Geometry: final body of the model. Coordinates: model frame, mm. A direction names the side the tool comes from. Coordinates: 2 decimals unless noted, no trailing zeros. Loops run counter-clockwise (first coordinate to the right, second up) from the corner with the lowest first, then second, coordinate; pieces in that order, holes last. Notation, with made-up numbers: (49, -17) - (91, -17) arc R26 cw to (91, 1) - close; hole circle Ø2 at (81, 29). An arc over 180 degrees is marked (long way). Put each result on its own line as item: value. Start each with the question number.
1) Contact query for flat-ended pins moving along their axis: pin 1 Ø2 at (x, y) = (-2.5, -2) entering from -Z; pin 2 Ø3.5 at (x, y) = (0, 2) entering from +Z; pin 3 Ø2 at (y, z) = (2, 17.37) entering from -X; pin 4 Ø5.5 at (y, z) = (-1, 6.5) entering from +X. Output: stop coordinate, or through.
2) Material intervals for line 1 along X through (y, z) = (2, 6); line 2 along Z through (x, y) = (4.3, 2); line 3 along Y through (x, z) = (0, 14.1), sorted ascending. Write a range as from..to.
3) Section C-C on z = 12. Output: boundary loops of the cut face in (x, y).
4) Section A-A on z = 16. Output: boundary loops of the cut face in (x, y).
5) Section B-B on z = 6. Output: boundary loops of the cut face in (x, y).
6) Reachability of faces 1 (the cylindrical face through (-0.1, -6.25, 7.3)), 2 (the flat face through (4, 2, 16)), 3 (the flat face through (0, 2, 14)), 4 (the flat face through (2, -4.4, 16)), 5 (the flat face through (-4, 4, 13.5)) from +Z, -Z, +X, -X, +Y, -Y: full face, straight path, thin tool, end or side. Return the list, or none.
7) Draft query along Y for faces 6 (the cylindrical face through (0.1, 6.25, 7.3)), 7 (the cylindrical face through (6.466, -2.681, 1.113)), 8 (the flat face through (0, 2, 0.5)), 9 (the flat face through (-5.75, 0, 7)). Return one class per face: +Y half, -Y half, draft (parallel to the pull), parting line (faces both ways), or undercut.
```python
from build123d import *

# Parameters (mm, degrees)
F0_R      = 7
F1_DEPTH  = 2
F3_DEPTH  = 11
F4_R      = 3
F5_DEPTH  = 10
F7_DEPTH  = 1
F8_R      = 1
F9_DEPTH  = 0.2
F10_W     = 0.5
F10_H     = 3
F10_W_2   = 2.5
F10_H_2   = 0.5
F11_DEPTH = 4.5
F12_R     = 0.625
F13_DEPTH = 25
F14_R     = 0.5
F15_DEPTH = 11.401
F16_R     = 1
F17_DEPTH = 9.5
F18_R     = 0.25


with BuildPart() as f1:
    # F0 (on Top) → F1 (new body)
    with BuildSketch(Plane.XY):
        Circle(F0_R)
    extrude(amount=F1_DEPTH)

    # F2 (on face) → F3 (join)
    with BuildSketch(Plane.XY.offset(2)):
        with BuildLine():
            Line((-5.75, 2.44949), (-5.75, -2.44949))
            ThreePointArc((-5.75, -2.44949), (0, -6.25), (5.75, -2.44949))
            Line((5.75, -2.44949), (5.75, 2.44949))
            ThreePointArc((5.75, 2.44949), (0, 6.25), (-5.75, 2.44949))
        make_face()
    extrude(amount=F3_DEPTH)

    # F4 (on face) → F5 (cut)
    with BuildSketch(Plane(origin=(0, 0, 0), x_dir=(1, 0, 0), z_dir=(0, 0, -1))):
        with Locations((0, -2)):
            Circle(F4_R)
    extrude(amount=-F5_DEPTH, mode=Mode.SUBTRACT)

    # F6 (on face) → F7 (join)
    with BuildSketch(Plane.XY.offset(13)):
        Polygon((-3.5, -4.5), (3.5, -4.5), (4.5, -3.5), (4.5, 3.5), (3.5, 4.5), (-3.5, 4.5), (-4.5, 3.5), (-4.5, -3.5), align=None)
    extrude(amount=F7_DEPTH)

    # F8 (on face) → F9 (join)
    with BuildSketch(Plane.XY.offset(14)):
        with BuildLine():
            Line((4.5, 0), (4.5, 4))
            Line((4.5, 4), (0, 4))
            ThreePointArc((0, 4), (-1.414214, 3.414214), (-2, 2))
            ThreePointArc((-2, 2), (-1.414214, 0.585786), (0, 0))
            Line((0, 0), (4.5, 0))
        make_face()
        with Locations((0, 2)):
            Circle(F8_R, mode=Mode.SUBTRACT)
    extrude(amount=F9_DEPTH)

    # F10 (on face) → F11 (join)
    with BuildSketch(Plane.XY.offset(14)):
        with Locations((4.25, 2)):
            Rectangle(F10_W, F10_H)
        with Locations((2.05, -4.15)):
            Rectangle(F10_W_2, F10_H_2)
        with Locations((-2.65, -1.25)):
            Rectangle(F10_W_2, F10_H_2)
    extrude(amount=F11_DEPTH)

    # F12 (on face) → F13 (cut)
    with BuildSketch(Plane.YZ.offset(4.5)):
        with Locations((2, 17.372569)):
            Circle(F12_R)
        with BuildLine():
            ThreePointArc((0.5, 17.372569), (1.06177, 18.186716), (2, 18.5))
            Line((2, 18.5), (0.5, 18.5))
            Line((0.5, 18.5), (0.5, 17.372569))
        make_face()
        with BuildLine():
            ThreePointArc((2, 18.5), (2.93823, 18.186716), (3.5, 17.372569))
            Line((3.5, 17.372569), (3.5, 18.5))
            Line((3.5, 18.5), (2, 18.5))
        make_face()
    extrude(amount=-F13_DEPTH, mode=Mode.SUBTRACT)

    # F14 (on face) → F15 (cut, through all)
    with BuildSketch(Plane.XZ.offset(4.4)):
        with Locations((2.05, 17.5)):
            Circle(F14_R)
        with BuildLine():
            ThreePointArc((2.05, 18.5), (2.850391, 18.219238), (3.3, 17.5))
            Line((3.3, 17.5), (3.3, 18.5))
            Line((3.3, 18.5), (2.05, 18.5))
        make_face()
        with BuildLine():
            ThreePointArc((0.8, 17.5), (1.249609, 18.219238), (2.05, 18.5))
            Line((2.05, 18.5), (0.8, 18.5))
            Line((0.8, 18.5), (0.8, 17.5))
        make_face()
        with Locations((-2.65, 17.5)):
            Circle(F14_R)
        with BuildLine():
            Line((-3.9, 18.5), (-3.9, 17.5))
            ThreePointArc((-3.9, 17.5), (-3.450391, 18.219238), (-2.65, 18.5))
            Line((-2.65, 18.5), (-3.9, 18.5))
        make_face()
        with BuildLine():
            ThreePointArc((-2.65, 18.5), (-1.849609, 18.219238), (-1.4, 17.5))
            Line((-1.4, 17.5), (-1.4, 18.5))
            Line((-1.4, 18.5), (-2.65, 18.5))
        make_face()
    extrude(amount=-F15_DEPTH, mode=Mode.SUBTRACT)

    # F16 (on face) → F17 (join)
    with BuildSketch(Plane(origin=(0, 0, 10), x_dir=(1, 0, 0), z_dir=(0, 0, -1))):
        with Locations((0, -2)):
            Circle(F16_R)
    extrude(amount=F17_DEPTH)

    # F18
    f18_edges = [f1.edges().sort_by_distance(p)[0] for p in [
        (-1, 2, 0.5),
        (-7, 0, 0),
        (0, 6.25, 13),
        (5.75, 0, 13),
        (0, -6.25, 13),
        (-5.75, 0, 13),
    ]]
    fillet(f18_edges, radius=F18_R)


solid = f1.part
```
Answer block:
1. pin 1: stops at z = 0
1. pin 2: stops at z = 14.2
1. pin 3: stops at x = 4
1. pin 4: stops at x = 5.75
2. line 1: x = -5.75..-3, -1..1, 3..5.75
2. line 2: z = 0..16.75, 18..18.5
2. line 3: y = 0..1, 3..4
3. outline: (-5.75, -2.45) arc R6.25 ccw to (5.75, -2.45) - (5.75, 2.45) arc R6.25 ccw to (-5.75, 2.45) - close
4. outline: (-3.9, -1.5) - (-1.4, -1.5) - (-1.4, -1) - (-3.9, -1) - close; (0.8, -4.4) - (3.3, -4.4) - (3.3, -3.9) - (0.8, -3.9) - close; (4, 0.5) - (4.5, 0.5) - (4.5, 3.5) - (4, 3.5) - close
5. outline: (-5.75, -2.45) arc R6.25 ccw to (5.75, -2.45) - (5.75, 2.45) arc R6.25 ccw to (-5.75, 2.45) - close; circle Ø2 at (0, 2); hole circle Ø6 at (0, 2)
6. face 1: +Z, -Y
6. face 2: +Z, -X, +Y, -Y
6. face 3: +Z
6. face 4: +Z, +X, -X, -Y
6. face 5: +Z, -X, +Y
7. face 6: +Y half
7. face 7: parting line
7. face 8: undercut
7. face 9: draft
